Read the model definition and answer for the solid it produces. Units are mm, in the model's axes. A direction names the side the tool comes from. Coordinates: 2 decimals unless noted, no trailing zeros. Write each loop counter-clockwise with the first axis right and the second up, starting at its lowest first coordinate (ties: lowest second). Pieces come first, ordered by that corner, then holes.
from build123d import *

# Parameters (mm, degrees)
F1_DEPTH = 300


with BuildPart() as f1:
    # F0 (on Top) → F1 (new body)
    with BuildSketch(Plane.XY):
        with BuildLine():
            ThreePointArc((0, 360.696902), (-305.348451, 55.348451), (0, -250))
            ThreePointArc((0, -250), (85.505036, -234.923155), (160.696902, -191.511111))
            Line((160.696902, -191.511111), (160.696902, -230))
            Line((160.696902, -230), (360.696902, -230))
            Line((360.696902, -230), (360.696902, 0))
            ThreePointArc((360.696902, 0), (255.051226, 255.051226), (0, 360.696902))
        make_face()
    extrude(amount=-F1_DEPTH)


solid = f1.part
Item 1: Determine the mould class of faces 3 (the cylindrical face through (-305.275, 62.063, -147.9)), 4 (the cylindrical face through (257.84, 252.23, -147.9)), 5 (the flat face through (23, 60, -300)), 6 (the flat face through (160.697, -210, -148)) for opening direction X: +X half, -X half, draft (parallel to the pull), parting line (faces both ways), or undercut.
Item 2: Find the intervals of material crossed by probe 1 along X at (y, z) = (-223.5, -22); probe 2 along X at (y, z) = (-195.5, -223.5); probe 3 along Y at (x, z) = (102.5, -169), in increasing order.
Item 3: The part is cut by section B-B (y = 247). Give the vertices of the cut face in (x, z).
Item 4: For faces 1 (the flat face through (259, -230, -148)), 2 (the flat face through (23, 60, 0)), determine the directions among +Z, -Z, +X, -X, +Y, -Y from which every point of the face is accessible in a straight line to the end or side of a thin tool.
Item 5: Given pin 1 (1 mm diameter, centred on y = -46.5, z = -49, fed in from -X); pin 2 (5 mm diameter, centred on x = -130, y = -69, fed in from +Z); pin 3 (3 mm diameter, centred on x = -197, z = -168.5, fed in from -Y); pin 4 (2 mm diameter, centred on x = -61, z = -206.5, fed in from +Y), each flat-ended and moving along its own axis, determine where each tip first touches the part or whether it passes through.
Item 6: The part is cut by section A-A (z = -77.5). Give the vertices of the cut face in (x, y), and give its area (3 significant figures).
Item 7: The part is cut by section C-C (x = 265). Give the vertices of the cut face in (y, z), and give its area (3 significant figures).
Answer:
1. face 3: -X half
1. face 4: +X half
1. face 5: draft
1. face 6: undercut
2. probe 1: x = -124.42 to 112.02, 160.7 to 360.7
2. probe 2: x = -174.11 to 155.82, 160.7 to 360.7
2. probe 3: y = -228.02 to 345.83
3. outline: (-237.71, -300) - (262.86, -300) - (262.86, 0) - (-237.71, 0) - close
4. face 1: +Z, -Z, +X, -Y
4. face 2: +Z, +X, -X, +Y, -Y
5. pin 1: stops at x = -288.04
5. pin 2: stops at z = 0
5. pin 3: stops at y = -179.21
5. pin 4: stops at y = 354.74
6. outline: (0, -250) arc R250 ccw to (160.7, -191.51) - (160.7, -230) - (360.7, -230) - (360.7, 0) arc R360.7 ccw to (0, 360.7) arc R305.35 ccw to start
6. area: 332,000 mm2
7. outline: (-230, -300) - (244.7, -300) - (244.7, 0) - (-230, 0) - close
7. area: 142,000 mm2
